Read the model definition and answer for the solid it produces. Units are mm, in the model's axes. Coordinates: 2 decimals unless noted, no trailing zeros. Loops run counter-clockwise (first coordinate to the right, second up) from the corner with the lowest first, then second, coordinate; pieces in that order, holes last. Notation, with made-up numbers: (-32.75, 61.5) -> (-2.75, 61.5) arc R23 cw to (-2.75, 69.5) -> close; hole circle Ø7 at (88.25, 35.5). An arc over 180 degrees is marked (long way). Answer as a JSON object with one key per item and string values. Group by question number.
1) Section B-B, the plane y = 0 is taken. Give the vertices of the cut face in (x, z), plus the area to 3 significant figures.
2) Consider probe 1 along Y at (x, z) = (0, 0.75); probe 2 along X at (y, z) = (-0.75, 2.25); probe 3 along X at (y, z) = (-1, 1). Determine where each line is inside the solid, lowest interval first. Write a range as [from, to].
3) Section C-C, the plane x = -3 is taken. Give the vertices of the cut face in (y, z).
4) Section A-A, the plane x = 0 is taken. Give the vertices of the cut face in (y, z), plus the area to 3 significant figures.
5) Determine the mould class of faces 1 (the face through (1.27, -3.07, 3.13)), 2 (the face through (3, -3, 6.35)), 3 (the face through (11.923, -3.755, 3.131)) for opening direction Y: released by +Y, released by -Y, zero draft, split by the parting line, or undercut.
6) Section D-D, the plane z = 4.5 is taken. Give the vertices of the cut face in (x, y).
7) A flat-ended cylindrical pin translates along its axis: P1, Ø2, axis at x = -7.94, y = 0, coming from the -Z side. Find the tip coordinate at first contact, or state that the pin passes through.
Autodesk Inventor part; units mm, degrees
ref_plane "YZ Plane" through (0, 0, 0) normal (1, 0, 0) x (0, 1, 0)
ref_plane "XZ Plane" through (0, 0, 0) normal (0, 1, 0) x (-1, 0, 0)
ref_plane "XY Plane" through (0, 0, 0) normal (0, 0, 1) x (1, 0, 0)
sketch "Sketch1" plane through (0, 0, 0) normal (0, 0, 1) x (1, 0, 0)
  circle A0 centre (0, 0) radius 12.5
  dimension "d0" = 25
extrude "Extrusion1" add sketch "Sketch1" along normal blind 6.35
sketch "Sketch2" plane through (0, 0, 6.35) normal (0, 0, 1) x (1, 0, 0)
  circle A0 centre (0, 0) radius 12.5
hole "Hole1" at (0, 0, 6.35) direction (0, 0, -1) diameter 6.647 end through all
sketch "Sketch3" plane through (0, 0, 6.35) normal (0, 0, 1) x (1, 0, 0)
  line L0 (-7.9375, 0) -> (7.9375, 0) construction
  point P0 (0, 0)
  point P1 (0, 0)
  dimension "d10" = 15.875
hole "Hole2" at (-7.9375, 0, 6.35) at (7.9375, 0, 6.35) direction (0, 0, -1) diameter 3.5 end through all
properties part number "Spanner Nut"
Determined:
{
 "1": {"outline": "(-12.5, 0) -> (-9.69, 0) -> (-9.69, 6.35) -> (-12.5, 6.35) -> close; (-6.19, 0) -> (-3.32, 0) -> (-3.32, 6.35) -> (-6.19, 6.35) -> close; (3.32, 0) -> (6.19, 0) -> (6.19, 6.35) -> (3.32, 6.35) -> close; (9.69, 0) -> (12.5, 0) -> (12.5, 6.35) -> (9.69, 6.35) -> close", "area": "72.1 mm²"},
 "2": {"probe 1": "[-12.5, -3.32], [3.32, 12.5]", "probe 2": "[-12.48, -9.52], [-6.36, -3.24], [3.24, 6.36], [9.52, 12.48]", "probe 3": "[-12.46, -9.37], [-6.5, -3.17], [3.17, 6.5], [9.37, 12.46]"},
 "3": {"outline": "(-12.13, 0) -> (-1.43, 0) -> (-1.43, 6.35) -> (-12.13, 6.35) -> close; (1.43, 0) -> (12.13, 0) -> (12.13, 6.35) -> (1.43, 6.35) -> close"},
 "4": {"outline": "(-12.5, 0) -> (-3.32, 0) -> (-3.32, 6.35) -> (-12.5, 6.35) -> close; (3.32, 0) -> (12.5, 0) -> (12.5, 6.35) -> (3.32, 6.35) -> close", "area": "117 mm²"},
 "5": {"face 1": "undercut", "face 2": "zero draft", "face 3": "split by the parting line"},
 "6": {"outline": "circle Ø25 at (0, 0); hole circle Ø3.5 at (-7.94, 0); hole circle Ø6.65 at (0, 0); hole circle Ø3.5 at (7.94, 0)"},
 "7": {"P1": "through"}
}
